Answer from the drawing. Dimensions are ordinates in mm from the lowest x, y and z of the part. Coordinates: 2 decimals unless noted, no trailing zeros. Order: outer loops, then holes, each group sorted by start corner. A loop starts at its lowest first (then second) coordinate and runs counter-clockwise, first axis right, second up. Notation, with made-up numbers: M 64,16.5 L 76,16.5 A8 cw 76,25.5 Z; hole C 74.5,85 d2. An arc over 180 degrees is marked long. Use a Markdown table: item, result.
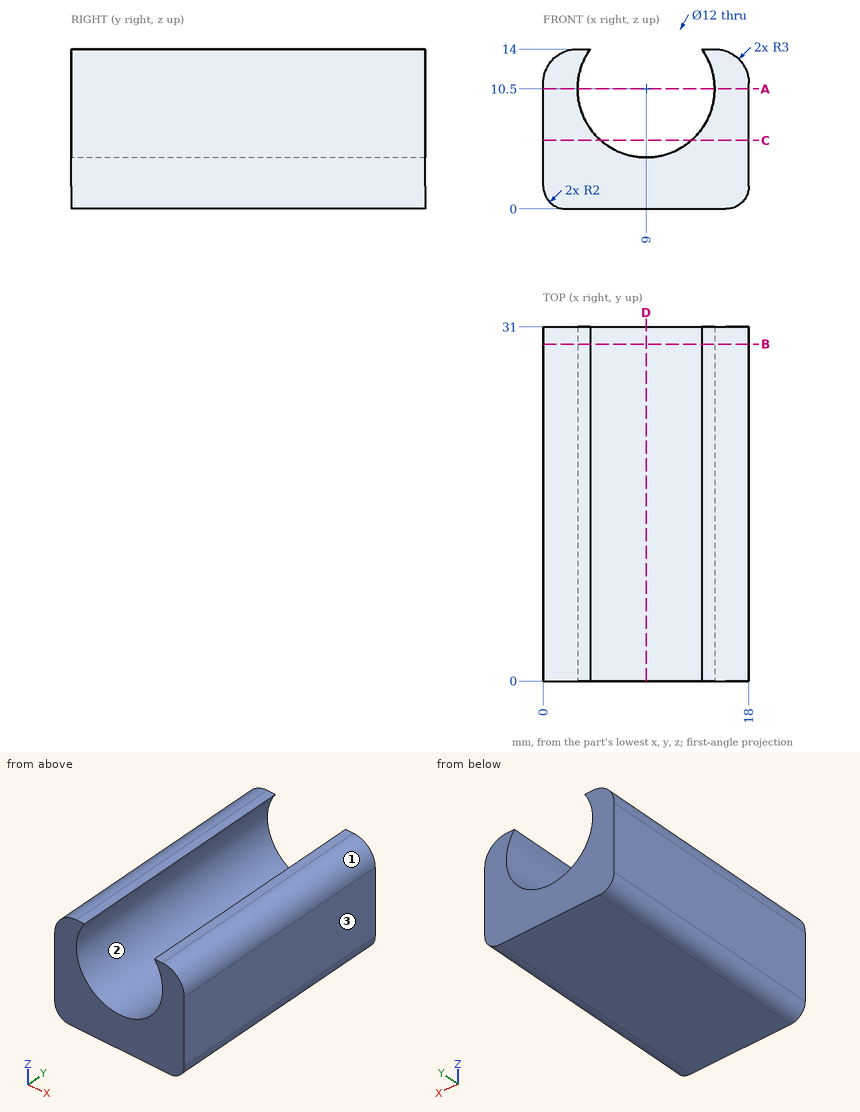
(1) A cutting plane is placed at A-A (z = 10.5). Determine the outline of the cut face in (x, y), then the cut area to 3 significant figures.
Conclusion:
| item | result |
|---|---|
| outline | M 0,0 L 3,0 L 3,31 L 0,31 Z; M 15,0 L 18,0 L 18,31 L 15,31 Z |
| area | 186 mm2 |
(2) A cutting plane is placed at B-B (y = 29.5). Determine the outline of the cut face in (x, z), then the cut area to 3 significant figures.
Conclusion:
| item | result |
|---|---|
| outline | M 0,2 A2 ccw 2,0 L 16,0 A2 ccw 18,2 L 18,11 A3 ccw 15,14 L 13.87,14 A6 cw long 4.13,14 L 3,14 A3 ccw 0,11 Z |
| area | 150 mm2 |
(3) Determine the mould class of the marked faces 1, 2 and 3 for opening direction Z: pulls with the +Z half, pulls with the -Z half, needs draft (parallel to the pull), parting line crosses it, or undercut.
Conclusion:
| item | result |
|---|---|
| face 1 | pulls with the +Z half |
| face 2 | undercut |
| face 3 | needs draft |
(4) Given P1, Ø6, axis at x = 9.5, y = 10, coming from the +Z side, flat-ended and moving along its own axis, determine where the tip first touches the part or whether it passes through.
Conclusion:
| item | result |
|---|---|
| P1 | z = 5.63 |
(5) A cutting plane is placed at C-C (z = 6). Determine the outline of the cut face in (x, y).
Conclusion:
| item | result |
|---|---|
| outline | M 0,0 L 5.03,0 L 5.03,31 L 0,31 Z; M 12.97,0 L 18,0 L 18,31 L 12.97,31 Z |
(6) Straight lines are drawn through the part: L1, parallel to X at y = 23.5, z = 10.5; L2, parallel to Z at x = 9, y = 25.5; L3, parallel to X at y = 15.5, z = 11.5. For each, find the intervals that lie inside material, in ascending order.
Conclusion:
| item | result |
|---|---|
| L1 | 0 to 3, 15 to 18 |
| L2 | 0 to 4.5 |
| L3 | 0.04 to 3.08, 14.92 to 17.96 |
(7) A cutting plane is placed at D-D (x = 9). Determine the outline of the cut face in (y, z), then the cut area to 4 significant figures.
Conclusion:
| item | result |
|---|---|
| outline | M 0,0 L 31,0 L 31,4.5 L 0,4.5 Z |
| area | 139.5 mm2 |
